Verification items for the finished model (mm, model axes). Face numbers are marked on the shaded views. A direction names the side the tool comes from. Coordinates: 2 decimals unless noted, no trailing zeros. Write each loop counter-clockwise with the first axis right and the second up, starting at its lowest first coordinate (ties: lowest second). Pieces come first, ordered by that corner, then holes.
```python
from build123d import *

# Parameters (mm, degrees)
F0_R     = 4
F1_DEPTH = 4
F2_R     = 2
F3_DEPTH = 6
F4_W     = 0.8
F4_H     = 3.919184
F5_DEPTH = 4


with BuildPart() as f1:
    # F0 (on Top) → F1 (new body)
    with BuildSketch(Plane.XY):
        with Locations((-51.708624, -21.201266)):
            Circle(F0_R)
    extrude(amount=F1_DEPTH)

    # F2 (on face) → F3 (join)
    with BuildSketch(Plane.XY.offset(4)):
        with Locations((-51.708624, -21.201266)):
            Circle(F2_R)
    extrude(amount=F3_DEPTH)

    # F4 (on face) → F5 (join)
    with BuildSketch(Plane.XY.offset(10)):
        with Locations((-51.708624, -21.201266)):
            Rectangle(F4_W, F4_H)
    extrude(amount=F5_DEPTH)


solid = f1.part
```
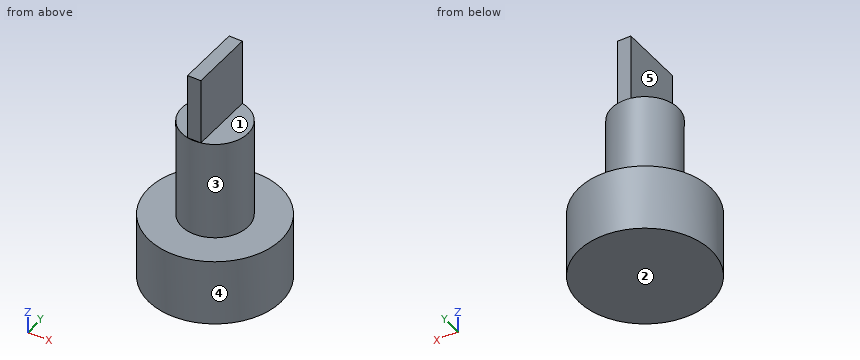
1. Tool access check on the marked faces 1, 2 and 3. Record the directions out of +Z, -Z, +X, -X, +Y, -Y that give a thin tool (end or side, any length) a straight path to the whole face; none if there is none.
2. Sectioned sample at B-B, the plane y = -22. Record the boundary of the cut face in (x, z), and give its area (3 significant figures).
3. Sectioned sample at D-D, the plane x = -50. Record the boundary of the cut face in (y, z), and give its area (3 significant figures).
4. Sectioned sample at C-C, the plane z = 12. Record the boundary of the cut face in (x, y), and give its area (3 significant figures).
5. Material ranges on L1, parallel to Z at x = -48.25, y = -20.5; L2, parallel to X at y = -22.5, z = 13; L3, parallel to Z at x = -52.5, y = -19.75, recorded low to high.
6. Draft check along Y on the marked faces 4 and 5. Enter one of: pulls with the +Y half, pulls with the -Y half, needs draft (parallel to the pull), parting line crosses it, or undercut.
7. Gauge pin test, flat ends, axial feed: P1, Ø3, axis at y = -21.5, z = 12, coming from the +X side; P2, Ø2, axis at x = -53.5, z = 4, coming from the -Y side; P3, Ø0.8, axis at x = -50.5, y = -20.5, coming from the +Z side. Record the tip position at first contact, or that the pin passes through.
8. Sectioned sample at A-A, the plane x = -53.5. Record the boundary of the cut face in (y, z).
Outcome:
1. face 1: +Z, +X, +Y, -Y
1. face 2: -Z, +X, -X, +Y, -Y
1. face 3: +Z
2. outline: (-55.63, 0) - (-47.79, 0) - (-47.79, 4) - (-49.88, 4) - (-49.88, 10) - (-51.31, 10) - (-51.31, 14) - (-52.11, 14) - (-52.11, 10) - (-53.54, 10) - (-53.54, 4) - (-55.63, 4) - close
2. area: 56.6 mm2
3. outline: (-24.82, 0) - (-17.58, 0) - (-17.58, 4) - (-20.16, 4) - (-20.16, 10) - (-22.24, 10) - (-22.24, 4) - (-24.82, 4) - close
3. area: 41.4 mm2
4. outline: (-52.11, -23.16) - (-51.31, -23.16) - (-51.31, -19.24) - (-52.11, -19.24) - close
4. area: 3.14 mm2
5. L1: z = 0 to 4
5. L2: x = -52.11 to -51.31
5. L3: z = 0 to 10
6. face 4: parting line crosses it
6. face 5: needs draft
7. P1: stops at x = -51.31
7. P2: stops at y = -25.12
7. P3: stops at z = 10
8. outline: (-24.78, 0) - (-17.62, 0) - (-17.62, 4) - (-20.31, 4) - (-20.31, 10) - (-22.09, 10) - (-22.09, 4) - (-24.78, 4) - close
